Autodesk Inventor part; units mm, degrees
ref_plane "YZ Plane" through (0, 0, 0) normal (1, 0, 0) x (0, 1, 0)
ref_plane "XZ Plane" through (0, 0, 0) normal (0, 1, 0) x (-1, 0, 0)
ref_plane "XY Plane" through (0, 0, 0) normal (0, 0, 1) x (1, 0, 0)
sketch "Skizze1" plane through (0, 0, 0) normal (0, 0, 1) x (1, 0, 0)
  line L0 (-64.5, 64.5) -> (64.5, 64.5)
  line L1 (64.5, 64.5) -> (64.5, -64.5)
  line L2 (64.5, -64.5) -> (-64.5, -64.5)
  line L3 (-64.5, -64.5) -> (-64.5, 64.5)
  line L4 (-64.5, 64.5) -> (64.5, -64.5) construction
  line L5 (64.5, 64.5) -> (-64.5, -64.5) construction
  point P0 (0, 0)
  dimension "d0" = 129
  dimension "d1" = 129
extrude "Extrusion1" add sketch "Skizze1" along normal blind 2
sketch "Skizze2" plane through (0, 0, 2) normal (0, 0, 1) x (1, 0, 0)
  line L0 (64.5, 64.5) -> (-64.5, 64.5)
  line L1 (-64.5, -64.5) -> (64.5, -64.5)
  line L2 (-64.5, 64.5) -> (64.5, 64.5)
  line L3 (64.5, 64.5) -> (64.5, -64.5)
  line L4 (64.5, -64.5) -> (-64.5, -64.5)
  line L5 (-64.5, -64.5) -> (-64.5, 64.5)
  line L6 (62.5, -47.5) -> (62.5, 47.5)
  line L7 (47.5, 62.5) -> (-47.5, 62.5)
  line L8 (-62.5, 47.5) -> (-62.5, -47.5)
  line L9 (-47.5, -62.5) -> (47.5, -62.5)
  line L10 (-47.5, 62.5) -> (-47.5, 57.5)
  line L11 (-57.5, 47.5) -> (-62.5, 47.5)
  line L12 (47.5, 62.5) -> (47.5, 57.5)
  line L13 (57.5, 47.5) -> (62.5, 47.5)
  line L14 (62.5, -47.5) -> (57.5, -47.5)
  line L15 (47.5, -57.5) -> (47.5, -62.5)
  line L16 (-62.5, -47.5) -> (-57.5, -47.5)
  line L17 (-47.5, -57.5) -> (-47.5, -62.5)
  arc A0 (-57.5, 47.5) -> (-47.5, 57.5) centre (-57.5, 57.5) ccw
  arc A1 (47.5, 57.5) -> (57.5, 47.5) centre (57.5, 57.5) ccw
  arc A2 (57.5, -47.5) -> (47.5, -57.5) centre (57.5, -57.5) ccw
  arc A3 (-47.5, -57.5) -> (-57.5, -47.5) centre (-57.5, -57.5) ccw
  point P0 (0, 0)
  point P1 (47.5, 47.5)
  point P2 (47.5, -47.5)
  point P3 (-47.5, -47.5)
  dimension "d4" = 2
  dimension "d5" = 17
  dimension "d8" = 10
  dimension "d9" = 2
  dimension "d10" = 2
  dimension "d11" = 2
extrude "Extrusion2" add sketch "Skizze2" along normal blind 20
sketch "Skizze3" plane through (0, 0, 2) normal (0, 0, 1) x (1, 0, 0)
  line L0 (-45, 38) -> (45, 38)
  line L1 (45, 38) -> (45, -38)
  line L2 (45, -38) -> (-45, -38)
  line L3 (-45, -38) -> (-45, 38)
  line L4 (-45, 38) -> (45, -38) construction
  line L5 (45, 38) -> (-45, -38) construction
  line L6 (64.5, 64.5) -> (-64.5, 64.5)
  line L7 (0, 64.5) -> (0, 45)
  line L8 (0, -45) -> (0, -64.5)
  line L9 (-64.5, -64.5) -> (64.5, -64.5)
  point P0 (0, 0)
  point P1 (45, 0)
  point P2 (-45, 0)
  dimension "d14" = 76
  dimension "d15" = 90
  dimension "d16" = 90
hole "Bohrung1" at (-45, 38, 2) at (45, 38, 2) at (45, 0, 2) at (45, -38, 2) at (-45, -38, 2) at (-45, 0, 2) at (0, 45, 2) at (0, -45, 2) direction (0, 0, -1) diameter 3 end through all
properties part number "Gehäuse_Sensor_Dummy"
Could you check a few things on this model? Use its own coordinates, in mm. A direction names the side the tool comes from. Give positions to 0.01 mm unless a question says otherwise; leave off trailing zeros. Order: outer loops, then holes, each group sorted by start corner. A loop starts at its lowest first (then second) coordinate and runs counter-clockwise, first axis right, second up.
Item 1: If we mould it in two halves opening along X, with no side actions, what happens to faces 3 (the face through (-64.5, -1, 11)), 4 (the face through (-1, -62.5, 12)), 5 (the face through (64.5, 1, 11)), 6 (the face through (46.464, 38.325, 0.986))? For each: pulls with the +X half, pulls with the -X half, needs draft (parallel to the pull), parting line crosses it, or undercut.
Item 2: For faces 1 (the face through (1, 62.5, 12)), 2 (the face through (-1, 64.5, 11)), which set-ups out of +Z, -Z, +X, -X, +Y, -Y let a thin tool reach every point of the face, with its end or its side?
Item 3: If we section it at B-B, the plane z = 8.75: Write out the boundary of the cut face in (x, y), plus the area to 3 significant figures.
Item 4: If we section it at C-C, the plane x = 45: Write out the boundary of the cut face in (y, z).
Item 5: If we section it at A-A, the plane x = 0: Write out the boundary of the cut face in (y, z).
Item 6: I'm going to push flat-ended pins straight in: pin 1 (5 mm diameter, centred on x = 11.5, y = 50.5, fed in from +Z); pin 2 (2 mm diameter, centred on x = -50.5, y = 51.5, fed in from -Z). Where does each tip first touch, or does it pass through?
Item 7: I need wall thicknesses on line 1 (X direction, y = 38, z = 1.5); line 2 (Y direction, x = -45, z = 1.05). Which ranges of each line are inside material? Lowest first, please.
Item 8: If we section it at D-D, the plane y = 45: Write out the boundary of the cut face in (x, z).
Values:
1. face 3: pulls with the -X half
1. face 4: undercut
1. face 5: pulls with the +X half
1. face 6: undercut
2. face 1: +Z
2. face 2: +Z, -Z, +X, -X, +Y
3. outline: (-64.5, -64.5) - (64.5, -64.5) - (64.5, 64.5) - (-64.5, 64.5) - close; hole (-62.5, -47.5) - (-57.5, -47.5) arc R10 cw to (-47.5, -57.5) - (-47.5, -62.5) - (47.5, -62.5) - (47.5, -57.5) arc R10 cw to (57.5, -47.5) - (62.5, -47.5) - (62.5, 47.5) - (57.5, 47.5) arc R10 cw to (47.5, 57.5) - (47.5, 62.5) - (-47.5, 62.5) - (-47.5, 57.5) arc R10 cw to (-57.5, 47.5) - (-62.5, 47.5) - close
3. area: 1,830 mm2
4. outline: (-64.5, 0) - (-39.5, 0) - (-39.5, 2) - (-62.5, 2) - (-62.5, 22) - (-64.5, 22) - close; (-36.5, 0) - (-1.5, 0) - (-1.5, 2) - (-36.5, 2) - close; (1.5, 0) - (36.5, 0) - (36.5, 2) - (1.5, 2) - close; (39.5, 0) - (64.5, 0) - (64.5, 22) - (62.5, 22) - (62.5, 2) - (39.5, 2) - close
5. outline: (-64.5, 0) - (-46.5, 0) - (-46.5, 2) - (-62.5, 2) - (-62.5, 22) - (-64.5, 22) - close; (-43.5, 0) - (43.5, 0) - (43.5, 2) - (-43.5, 2) - close; (46.5, 0) - (64.5, 0) - (64.5, 22) - (62.5, 22) - (62.5, 2) - (46.5, 2) - close
6. pin 1: stops at z = 2
6. pin 2: stops at z = 0
7. line 1: x = -64.5 to -46.5, -43.5 to 43.5, 46.5 to 64.5
7. line 2: y = -64.5 to -39.5, -36.5 to -1.5, 1.5 to 36.5, 39.5 to 64.5
8. outline: (-64.5, 0) - (-1.5, 0) - (-1.5, 2) - (-62.5, 2) - (-62.5, 22) - (-64.5, 22) - close; (1.5, 0) - (64.5, 0) - (64.5, 22) - (62.5, 22) - (62.5, 2) - (1.5, 2) - close
